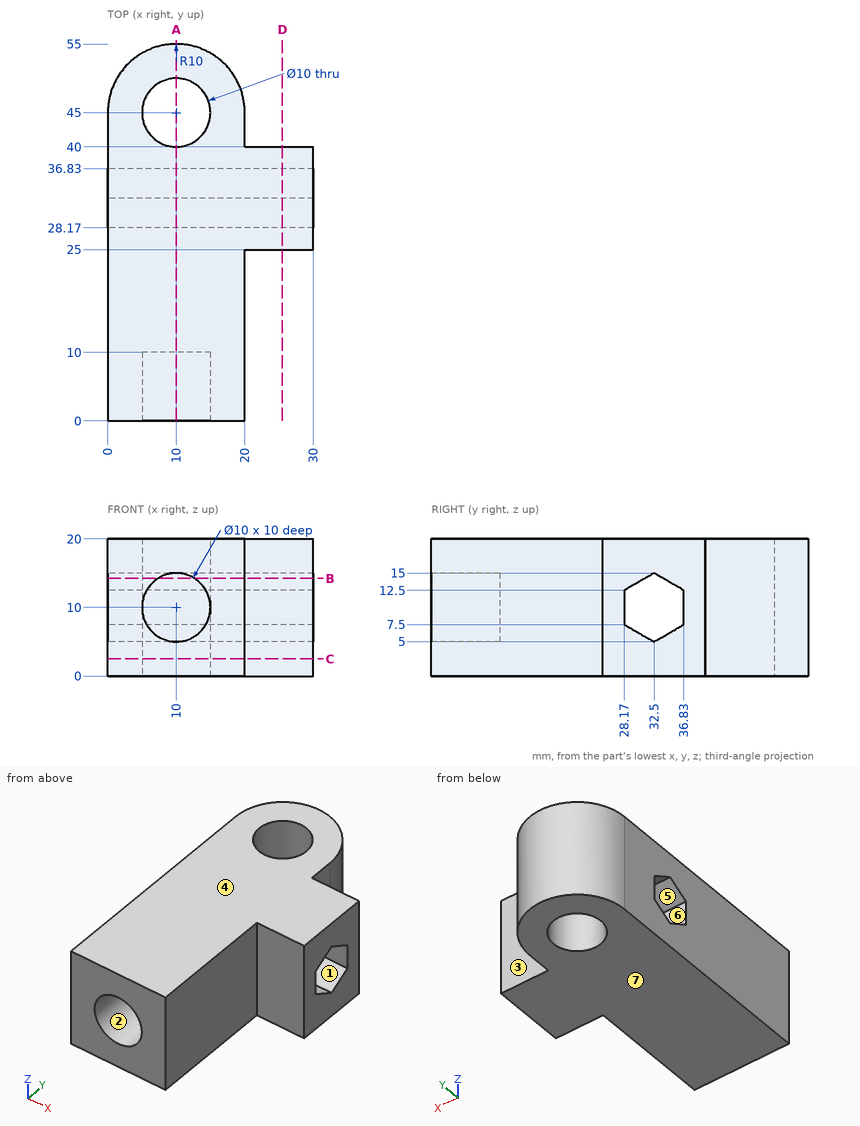
Job drawing, mm, ordinate dimensions from the low corner. One solid piece. A direction names the side the tool comes from. Give positions to 0.01 mm unless a question says otherwise; leave off trailing zeros. Write each loop counter-clockwise with the first axis right and the second up, starting at its lowest first coordinate (ties: lowest second). Pieces come first, ordered by that corner, then holes. Notation, with made-up numbers: (67, 17) - (107, 17) arc R21 cw to (107, 55) - close; hole circle Ø9 at (28.5, -20.75). An arc over 180 degrees is marked (long way). Answer as CSV lines item,"result".
1. Band-saw the part on A-A (x = 10). Write the cut outline in (y, z), and give its area (3 significant figures).
Responses:
outline,"(0, 0) - (40, 0) - (40, 20) - (0, 20) - (0, 15) - (10, 15) - (10, 5) - (0, 5) - close; (50, 0) - (55, 0) - (55, 20) - (50, 20) - close; hole (28.17, 7.5) - (32.5, 5) - (36.83, 7.5) - (36.83, 12.5) - (32.5, 15) - (28.17, 12.5) - close"
area,"735 mm2"
2. Band-saw the part on B-B (z = 14.25). Write the cut outline in (x, y).
Responses:
outline,"(0, 0) - (7.37, 0) - (7.37, 10) - (12.63, 10) - (12.63, 0) - (20, 0) - (20, 25) - (30, 25) - (30, 31.2) - (0, 31.2) - close; (0, 33.8) - (30, 33.8) - (30, 40) - (20, 40) - (20, 45) arc R10 ccw to (0, 45) - close; hole circle Ø10 at (10, 45)"
3. Band-saw the part on C-C (z = 2.5). Write the cut outline in (x, y).
Responses:
outline,"(0, 0) - (20, 0) - (20, 25) - (30, 25) - (30, 40) - (20, 40) - (20, 45) arc R10 ccw to (0, 45) - close; hole circle Ø10 at (10, 45)"
4. Two-plate mould, pull along Z, no slides. Class the marked faces 4, 5, 6 and 7: +Z half, -Z half, draft (parallel to the pull), parting line (faces both ways), or undercut.
Responses:
face 4,"+Z half"
face 5,"undercut"
face 6,"undercut"
face 7,"-Z half"
5. 3-axis set-ups, long thin cutter, end or side, ignore diameter. For the marked faces 1, 2 and 3: which of +Z, -Z, +X, -X, +Y, -Y reach the whole face in a straight line?
Responses:
face 1,"+X, -X"
face 2,"-Y"
face 3,"+Z, -Z, +X, +Y"
6. Drill centre lines: L1, parallel to Y at x = 10, z = 8.5; L2, parallel to Z at x = 10, y = 7.5; L3, parallel to Y at x = 10, z = 14.75. Where is each one in solid material? Low to high. Write a range as [from, to].
Responses:
L1,"y = [10, 28.17], [36.83, 40], [50, 55]"
L2,"z = [0, 5], [15, 20]"
L3,"y = [10, 32.07], [32.93, 40], [50, 55]"
7. Pin check, flat tips, straight feed: pin 1 (8 mm diameter, centred on y = 15, z = 14, fed in from +X); pin 2 (6 mm diameter, centred on x = 22.5, z = 2, fed in from -Y); pin 3 (5 mm diameter, centred on x = 6.5, z = 15.5, fed in from +Y); pin 4 (3 mm diameter, centred on x = 23.5, z = 9.5, fed in from +Y). Stop position of each tip, or through.
Responses:
pin 1,"stops at x = 20"
pin 2,"stops at y = 0"
pin 3,"stops at y = 54.95"
pin 4,"stops at y = 40"
8. Band-saw the part on D-D (x = 25.5). Write the cut outline in (y, z).
Responses:
outline,"(25, 0) - (40, 0) - (40, 20) - (25, 20) - close; hole (28.17, 7.5) - (32.5, 5) - (36.83, 7.5) - (36.83, 12.5) - (32.5, 15) - (28.17, 12.5) - close"
